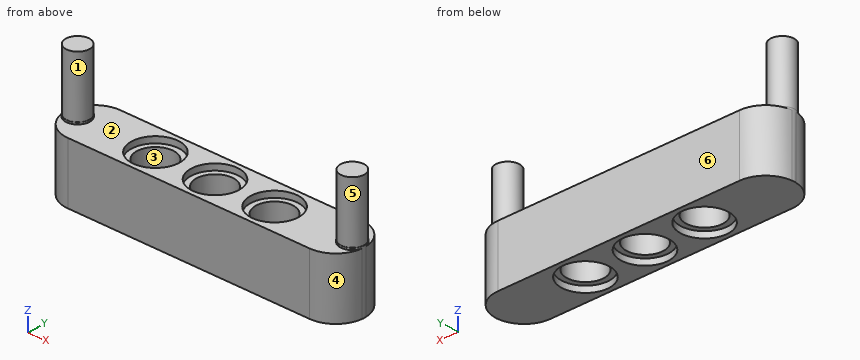
from build123d import *

# Parameters (mm, degrees)
SKETCH1_W                = 39
SKETCH1_H                = 7.38
BOSS_EXTRUDE1_DEPTH      = 7.76
SKETCH2_R                = 2.4
CUT_EXTRUDE1_DEPTH       = 7.76
CUT_EXTRUDE2_OUTLINE_R   = 3.1
CUT_EXTRUDE2_OUTLINE_R_2 = 2.4
CUT_EXTRUDE2_DEPTH       = 0.8
CUT_EXTRUDE3_START       = 6.96
CUT_EXTRUDE3_OUTLINE_R   = 3.1
CUT_EXTRUDE3_OUTLINE_R_2 = 2.4
CUT_EXTRUDE3_DEPTH       = 0.8
LPATTERN3_COUNT          = 3
LPATTERN3_PITCH          = 7.79
LPATTERN6_COUNT          = 3
LPATTERN6_PITCH          = 7.79
FILLET1_R                = 3.69
FILLET2_R                = 3.69
FILLET3_R                = 3.69
FILLET4_R                = 3.69
SKETCH3_R                = 3.1
BOSS_EXTRUDE2_DEPTH      = 7.76
BOSS_EXTRUDE3_START      = -7.76
SKETCH4_R                = 3.1
BOSS_EXTRUDE3_DEPTH      = 7.76
SKETCH11_R               = 1.525
BOSS_EXTRUDE7_DEPTH      = 8
SKETCH12_R               = 1.555
BOSS_EXTRUDE8_DEPTH      = 8
SKETCH14_R               = 1.555
BOSS_EXTRUDE9_DEPTH      = 8


# Read off the part's stored shape, not the designer's step: Cut-Extrude2, Cut-Extrude3
with BuildPart() as part:
    # Sketch1 → Boss-Extrude1 (new body)
    with BuildSketch(Plane.XY):
        with Locations((19.5, 3.69)):
            Rectangle(SKETCH1_W, SKETCH1_H)
    extrude(amount=BOSS_EXTRUDE1_DEPTH)

    # Sketch2 → Cut-Extrude1 (cut)
    with BuildSketch(Plane.XY.offset(7.76)):
        with Locations((19.5, 3.69)):
            Circle(SKETCH2_R)
    cut_extrude1 = extrude(amount=-CUT_EXTRUDE1_DEPTH, mode=Mode.SUBTRACT)

    # Cut-Extrude2 outline → Cut-Extrude2 (cut)
    with BuildSketch(Plane.XY):
        with Locations((19.5, 3.69)):
            Circle(CUT_EXTRUDE2_OUTLINE_R)
        with Locations((19.5, 3.69)):
            Circle(CUT_EXTRUDE2_OUTLINE_R_2, mode=Mode.SUBTRACT)
    cut_extrude2 = extrude(amount=CUT_EXTRUDE2_DEPTH, mode=Mode.SUBTRACT)

    # Cut-Extrude3 outline → Cut-Extrude3 (cut)
    with BuildSketch(Plane.XY.offset(CUT_EXTRUDE3_START)):
        with Locations((19.5, 3.69)):
            Circle(CUT_EXTRUDE3_OUTLINE_R)
        with Locations((19.5, 3.69)):
            Circle(CUT_EXTRUDE3_OUTLINE_R_2, mode=Mode.SUBTRACT)
    cut_extrude3 = extrude(amount=CUT_EXTRUDE3_DEPTH, mode=Mode.SUBTRACT)

    # LPattern3: Cut-Extrude1, Cut-Extrude2, Cut-Extrude3 ×3
    with Locations(*[(-i * LPATTERN3_PITCH, 0, 0) for i in range(1, LPATTERN3_COUNT)]):
        add(cut_extrude1, mode=Mode.SUBTRACT)
        add(cut_extrude2, mode=Mode.SUBTRACT)
        add(cut_extrude3, mode=Mode.SUBTRACT)

    # LPattern6: Cut-Extrude1, Cut-Extrude2, Cut-Extrude3 ×3
    with Locations(*[(i * LPATTERN6_PITCH, 0, 0) for i in range(1, LPATTERN6_COUNT)]):
        add(cut_extrude1, mode=Mode.SUBTRACT)
        add(cut_extrude2, mode=Mode.SUBTRACT)
        add(cut_extrude3, mode=Mode.SUBTRACT)

    # Fillet1
    fillet1_edges = [part.edges().sort_by_distance(p)[0] for p in [
        (0, 7.38, 3.88),
    ]]
    fillet(fillet1_edges, radius=FILLET1_R)

    # Fillet2
    fillet2_edges = [part.edges().sort_by_distance(p)[0] for p in [
        (0, 0, 3.88),
    ]]
    fillet(fillet2_edges, radius=FILLET2_R - 0.0001)  # a hair under: the kernel refuses the full size

    # Fillet3
    fillet3_edges = [part.edges().sort_by_distance(p)[0] for p in [
        (39, 7.38, 3.88),
    ]]
    fillet(fillet3_edges, radius=FILLET3_R)

    # Fillet4
    fillet4_edges = [part.edges().sort_by_distance(p)[0] for p in [
        (39, 0, 3.88),
    ]]
    fillet(fillet4_edges, radius=FILLET4_R - 0.0001)  # a hair under: the kernel refuses the full size

    # Sketch3 → Boss-Extrude2 (add)
    with BuildSketch(Plane(origin=(0, 0, 0), x_dir=(-1, 0, 0), z_dir=(0, 0, -1))):
        with Locations((-35.08, 3.69)):
            Circle(SKETCH3_R)
    extrude(amount=-BOSS_EXTRUDE2_DEPTH)

    # Sketch4 → Boss-Extrude3 (add)
    with BuildSketch(Plane.XY.offset(7.76).offset(BOSS_EXTRUDE3_START)):
        with Locations((3.92, 3.69)):
            Circle(SKETCH4_R)
    extrude(amount=BOSS_EXTRUDE3_DEPTH)

    # Sketch11 → Boss-Extrude7 (add)
    with BuildSketch(Plane.XY.offset(7.76)):
        with Locations(Location((1.54, 3.69, 0), (0, 0, 180))):
            Circle(SKETCH11_R)
        with Locations(Location((37.46, 3.69, 0), (0, 0, 180))):
            Circle(SKETCH11_R)
    extrude(amount=BOSS_EXTRUDE7_DEPTH)

    # Sketch12 → Boss-Extrude8 (add)
    with BuildSketch(Plane(origin=(0, 0, 0), x_dir=(-1, 0, 0), z_dir=(0, 0, -1))):
        with Locations((-37.46, 3.69)):
            Circle(SKETCH12_R)
    extrude(amount=-BOSS_EXTRUDE8_DEPTH)

    # Sketch14 → Boss-Extrude9 (add)
    with BuildSketch(Plane(origin=(0, 0, 0), x_dir=(-1, 0, 0), z_dir=(0, 0, -1))):
        with Locations((-1.54, 3.69)):
            Circle(SKETCH14_R)
    extrude(amount=-BOSS_EXTRUDE9_DEPTH)


solid = part.part
CAD build for the part. Positions are in the model's coordinates, mm. Face numbers are marked on the shaded views. A direction names the side the tool comes from. Give positions to 0.01 mm unless a question says otherwise; leave off trailing zeros. Write each loop counter-clockwise with the first axis right and the second up, starting at its lowest first coordinate (ties: lowest second). Pieces come first, ordered by that corner, then holes. Notation, with made-up numbers: (8.25, 59) -> (57.25, 59) arc R28 cw to (57.25, 85) -> close; hole circle Ø8 at (-12, -4). An arc over 180 degrees is marked (long way). Return JSON: item names as keys, results as strings.
Item 1: Drop flat-ended pins along their axis: pin 1 (2 mm diameter, centred on x = 9, y = 6, fed in from +Z); pin 2 (1 mm diameter, centred on y = 3, z = 7, fed in from +X); pin 3 (1.9 mm diameter, centred on x = 28, y = 5, fed in from +Z). Give the stop position or say it passes through.
Answer below:
{"pin 1": "stops at z = 7.76", "pin 2": "stops at x = 39", "pin 3": "stops at z = 6.96"}
Item 2: Band-saw the part on D-D (x = 26). List the corners of the cut face in (y, z), then the cut area to 3 significant figures.
Answer below:
{"outline": "(0, 0) -> (0.87, 0) -> (0.87, 0.8) -> (1.67, 0.8) -> (1.67, 6.96) -> (0.87, 6.96) -> (0.87, 7.76) -> (0, 7.76) -> close; (5.71, 0.8) -> (6.51, 0.8) -> (6.51, 0) -> (7.38, 0) -> (7.38, 7.76) -> (6.51, 7.76) -> (6.51, 6.96) -> (5.71, 6.96) -> close", "area": "23.3 mm2"}
Item 3: Band-saw the part on B-B (z = 10.5). List the corners of the cut face in (x, y) (3 decimals).
Answer below:
{"outline": "circle Ø3.05 at (1.54, 3.69); circle Ø3.05 at (37.46, 3.69)"}
Item 4: Two-plate mould, pull along Y, no slides. Class the marked faces 1, 2, 3 and 4: +Y half, -Y half, draft (parallel to the pull), parting line (faces both ways), or undercut.
Answer below:
{"face 1": "parting line", "face 2": "draft", "face 3": "undercut", "face 4": "-Y half"}
Item 5: Band-saw the part on A-A (x = 19.5). List the corners of the cut face in (y, z).
Answer below:
{"outline": "(0, 0) -> (0.59, 0) -> (0.59, 0.8) -> (1.29, 0.8) -> (1.29, 6.96) -> (0.59, 6.96) -> (0.59, 7.76) -> (0, 7.76) -> close; (6.09, 0.8) -> (6.79, 0.8) -> (6.79, 0) -> (7.38, 0) -> (7.38, 7.76) -> (6.79, 7.76) -> (6.79, 6.96) -> (6.09, 6.96) -> close"}
Item 6: Drill centre lines: probe 1 along Y at (x, z) = (27.29, 5); probe 2 along Y at (x, z) = (27.29, 0.45); probe 3 along Z at (x, y) = (33, 3.75). Where is each one in solid material? Low to high.
Answer below:
{"probe 1": "y = 0 to 1.29, 6.09 to 7.38", "probe 2": "y = 0 to 0.59, 6.79 to 7.38", "probe 3": "z = 0 to 7.76"}
Item 7: Tool access for the marked faces 5 and 6: list every direction of +Z, -Z, +X, -X, +Y, -Y with a clear straight run to the whole face (end or side of a thin tool).
Answer below:
{"face 5": "+Z", "face 6": "+Z, -Z, +X, -X, +Y"}
Item 8: Band-saw the part on C-C (z = 2.25). List the corners of the cut face in (x, y) (3 decimals).
Answer below:
{"outline": "(0.011, 3.408) arc R3.69 ccw to (3.69, 0) -> (35.31, 0) arc R3.69 ccw to (38.989, 3.408) arc R1.555 ccw to (38.989, 3.972) arc R3.69 ccw to (35.31, 7.38) -> (3.69, 7.38) arc R3.69 ccw to (0.011, 3.972) arc R1.555 ccw to start; hole circle Ø4.8 at (11.71, 3.69); hole circle Ø4.8 at (19.5, 3.69); hole circle Ø4.8 at (27.29, 3.69)"}
